Source: three-view drawing plus pictorial views. Frame: mm from the lowest corner of the part. A direction names the side the tool comes from. Give positions to 0.01 mm unless a question says otherwise; leave off trailing zeros. Write each loop counter-clockwise with the first axis right and the second up, starting at its lowest first coordinate (ties: lowest second). Pieces come first, ordered by that corner, then holes.
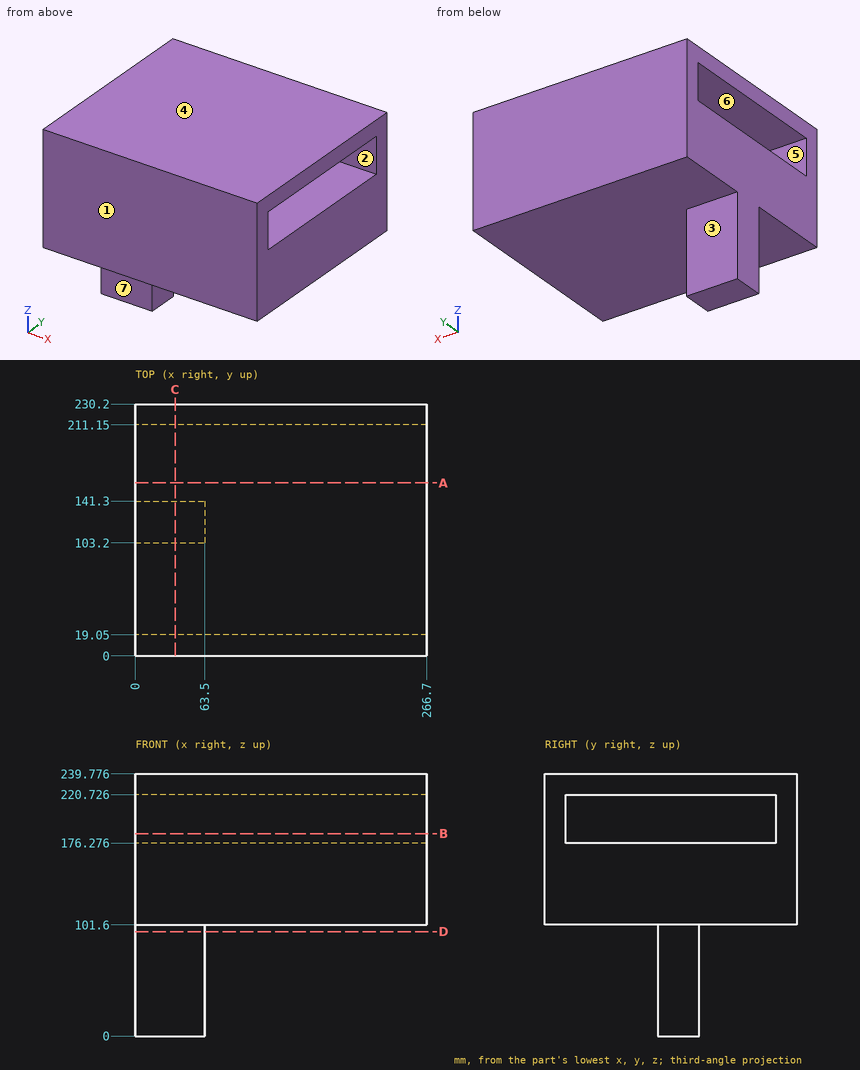
Q1. Pull-direction query (Z, two-part tool) for the marked faces 4, 5, 6 and 7; classes: released by +Z, released by -Z, zero draft, split by the parting line, or undercut.
Filled sheet:
face 4: released by +Z
face 5: undercut
face 6: undercut
face 7: zero draft
Q2. Ray query, line 1 along Z through (x, y) = (179, 118); line 2 along Y through (x, z) = (148.5, 180); line 3 along Z through (x, y) = (35, 122). Return the intervals inside material, ascending.
Filled sheet:
line 1: z = 101.6 to 176.28, 220.73 to 239.78
line 2: y = 0 to 19.05, 211.15 to 230.2
line 3: z = 0 to 176.28, 220.73 to 239.78
Q3. Section B-B on z = 185. Output: boundary loops of the cut face in (x, y).
Filled sheet:
outline: (0, 0) - (266.7, 0) - (266.7, 19.05) - (0, 19.05) - close; (0, 211.15) - (266.7, 211.15) - (266.7, 230.2) - (0, 230.2) - close
Q4. Section A-A on y = 158. Output: boundary loops of the cut face in (x, z).
Filled sheet:
outline: (0, 101.6) - (266.7, 101.6) - (266.7, 176.28) - (0, 176.28) - close; (0, 220.73) - (266.7, 220.73) - (266.7, 239.78) - (0, 239.78) - close
Q5. Pin query (flat end, axial travel): P1, Ø8, axis at x = 107.5, z = 179, coming from the -Y side. Return the tip coordinate at first contact, or that it passes through.
Filled sheet:
P1: stops at y = 0
Q6. Section D-D on z = 95.5. Output: boundary loops of the cut face in (x, y), plus the area to 3 significant figures.
Filled sheet:
outline: (0, 103.2) - (63.5, 103.2) - (63.5, 141.3) - (0, 141.3) - close
area: 2,420 mm2
Q7. Section C-C on x = 36.5. Output: boundary loops of the cut face in (y, z).
Filled sheet:
outline: (0, 101.6) - (103.2, 101.6) - (103.2, 0) - (141.3, 0) - (141.3, 101.6) - (230.2, 101.6) - (230.2, 239.78) - (0, 239.78) - close; hole (19.05, 176.28) - (211.15, 176.28) - (211.15, 220.73) - (19.05, 220.73) - close
Q8. Access query for the marked faces 1, 2 and 3. Directions: +Z, -Z, +X, -X, +Y, -Y. A direction counts if a zero-diameter tool reaches every point of the face in a straight line with its end or side. Return the directions, or none.
Filled sheet:
face 1: +Z, -Z, +X, -X, -Y
face 2: +X, -X
face 3: -Z, +X, -X, +Y
